```python
from build123d import *

# Parameters (mm, degrees)
SKETCH2_R           = 12
BOSS_EXTRUDE1_DEPTH = 86
SKETCH3_R           = 12.5
SKETCH3_R_2         = 6
BOSS_EXTRUDE2_DEPTH = 11


with BuildPart() as part:
    # Sketch1 → Revolve1 (revolve)
    with BuildSketch(Plane(origin=(0, 0, 0), x_dir=(1, 0, 0), z_dir=(0, 1, 0))):
        Polygon((0, 0), (0, 26.5), (2, 26.5), (2, 12), (122, 12), (122, 0), align=None)
    revolve(axis=Axis((122, 0, 0), (-1, 0, 0)))

    # Sketch2 → Boss-Extrude1 (add)
    with BuildSketch(Plane.ZY):
        Circle(SKETCH2_R)
    extrude(amount=BOSS_EXTRUDE1_DEPTH)

    # Sketch3 → Boss-Extrude2 (add, symmetric)
    with BuildSketch(Plane(origin=(0, 0, 0), x_dir=(1, 0, 0), z_dir=(0, 1, 0))):
        with Locations((-97, 0)):
            Circle(SKETCH3_R)
        with Locations((-97, 0)):
            Circle(SKETCH3_R_2, mode=Mode.SUBTRACT)
    extrude(amount=BOSS_EXTRUDE2_DEPTH, both=True)


solid = part.part
```
Check sheet for the modelled part. Datum: model origin and axes. Units: mm. A direction names the side the tool comes from. Give positions to 0.01 mm unless a question says otherwise; leave off trailing zeros. Write each loop counter-clockwise with the first axis right and the second up, starting at its lowest first coordinate (ties: lowest second). Pieces come first, ordered by that corner, then holes.
Item 1: Draft check along X on faces 1 (the face through (122, 0, 0)), 2 (the face through (-42.4, 0.53, -11.99)), 3 (the face through (-95, 11, -6)). Enter one of: released by +X, released by -X, zero draft, split by the parting line, or undercut.
Item 2: Cross-section at B-B (y = 0). Enter the section's corners in (x, z).
Item 3: Scan lines: L1, parallel to Z at x = -97, y = 5.25; L2, parallel to X at y = 9, z = 0.5; L3, parallel to X at y = 23.5, z = 0. Record each from-to range of solid material in increasing order.
Item 4: Gauge pin test, flat ends, axial feed: pin 1 (6 mm diameter, centred on x = -1.5, y = -5, fed in from +Z); pin 2 (6 mm diameter, centred on x = 18, y = -8, fed in from -Z); pin 3 (0.5 mm diameter, centred on y = -11.5, z = -2.5, fed in from -X); pin 4 (8 mm diameter, centred on x = 87, y = 17.5, fed in from +Z). Record the tip position at first contact, or that the pin passes through.
Item 5: Cross-section at C-C (x = -97). Enter the section's corners in (y, z), and give its area (3 significant figures).
Item 6: Cross-section at A-A (z = 0). Enter the section's corners in (x, y), and give its area (3 significant figures).
Item 7: Access from +Z, -Z, +X, -X, +Y, -Y to the whole of each face (thin tool, end or side, straight path). Record for faces 4 (the face through (1.014, -22.345, -14.246)), 5 (the face through (62.84, -0.53, 11.99)).
Item 8: Cross-section at D-D (x = -45). Enter the section's corners in (y, z).
Report:
1. face 1: released by +X
1. face 2: undercut
1. face 3: zero draft
2. outline: (-86, -12) - (0, -12) - (0, -26.5) - (2, -26.5) - (2, -12) - (122, -12) - (122, 12) - (2, 12) - (2, 26.5) - (0, 26.5) - (0, 12) - (-86, 12) - (-86, 5.94) arc R12.5 ccw (long way) to (-86, -5.94) - close; hole circle Ø12 at (-97, 0)
3. L1: z = -12.5 to -6, 6 to 12.5
3. L2: x = -109.49 to -102.98, -91.02 to 122
3. L3: x = 0 to 2
4. pin 1: stops at z = 26.39
4. pin 2: stops at z = -10.91
4. pin 3: stops at x = -86
4. pin 4: passes through
5. outline: (-11, -12.5) - (11, -12.5) - (11, -6) - (-11, -6) - close; (-11, 6) - (11, 6) - (11, 12.5) - (-11, 12.5) - close
5. area: 286 mm2
6. outline: (-109.5, -11) - (-103, -11) - (-103, 11) - (-109.5, 11) - close; (-91, -11) - (-86, -11) - (-86, -12) - (0, -12) - (0, -26.5) - (2, -26.5) - (2, -12) - (122, -12) - (122, 12) - (2, 12) - (2, 26.5) - (0, 26.5) - (0, 12) - (-86, 12) - (-86, 11) - (-91, 11) - close
6. area: 5,300 mm2
7. face 4: +X, -X
7. face 5: +X
8. outline: circle Ø24 at (0, 0)
